```python
from build123d import *

# Parameters (mm, degrees)
F4_DEPTH = 25.4
F5_W     = 25.4
F5_H     = 25.4
F6_DEPTH = 76.2
F7_W     = 25.4
F7_H     = 25.4
F8_DEPTH = 88.9


# Not quite as in the source:
# - a variable given as a bare number and used for a length is read in inches; the dataset says mm whatever the document's units were


with BuildPart() as f4:
    # F3 (on Front) → F4 (new body)
    with BuildSketch(Plane.XZ):
        Polygon((0, 25.4), (0, 0), (25.4, 0), (101.6, 0), (101.6, 25.4), (25.4, 25.4), (25.4, 63.5), (0, 63.5), align=None)
    extrude(amount=-F4_DEPTH)

    # F5 (on face) → F6 (join)
    with BuildSketch(Plane(origin=(0, 25.4, 0), x_dir=(-1, 0, 0), z_dir=(0, 1, 0))):
        with Locations((-12.7, 50.8)):
            Rectangle(F5_W, F5_H)
    extrude(amount=F6_DEPTH)

    # F7 (on face) → F8 (join)
    with BuildSketch(Plane(origin=(0, 25.4, 0), x_dir=(-1, 0, 0), z_dir=(0, 1, 0))):
        with Locations((-88.9, 12.7)):
            Rectangle(F7_W, F7_H)
    extrude(amount=F8_DEPTH)


solid = f4.part
```
Verification items for the finished model (mm, model axes). A direction names the side the tool comes from. Coordinates: 2 decimals unless noted, no trailing zeros. Loops run counter-clockwise (first coordinate to the right, second up) from the corner with the lowest first, then second, coordinate; pieces in that order, holes last. Notation, with made-up numbers: (26, -31.75) - (33, -31.75) arc R29 cw to (33, -3.75) - close; hole circle Ø2 at (69.5, -2.75). An arc over 180 degrees is marked (long way). Put each result on its own line as item: value.
Item 1: Section check A-A (y = 37). Enter the section's corners in (x, z), then the cut area to 3 significant figures.
Conclusion:
outline: (0, 38.1) - (25.4, 38.1) - (25.4, 63.5) - (0, 63.5) - close; (76.2, 0) - (101.6, 0) - (101.6, 25.4) - (76.2, 25.4) - close
area: 1,290 mm2
Item 2: Section check B-B (x = 13.5). Enter the section's corners in (y, z), then the cut area to 3 significant figures.
Conclusion:
outline: (0, 0) - (25.4, 0) - (25.4, 38.1) - (101.6, 38.1) - (101.6, 63.5) - (0, 63.5) - close
area: 3,550 mm2
Item 3: Section check D-D (y = 18.5). Enter the section's corners in (x, z), then the cut area to 3 significant figures.
Conclusion:
outline: (0, 0) - (101.6, 0) - (101.6, 25.4) - (25.4, 25.4) - (25.4, 63.5) - (0, 63.5) - close
area: 3,550 mm2
Item 4: Scan lines: line 1 along Z through (x, y) = (83.5, 9.5); line 2 along X through (y, z) = (59.5, 7.5). Record each from-to range of solid material in increasing order.
Conclusion:
line 1: z = 0 to 25.4
line 2: x = 76.2 to 101.6
Item 5: Gauge pin test, flat ends, axial feed: pin 1 Ø7.5 at (x, y) = (11.5, 67.5) entering from -Z; pin 2 Ø10 at (y, z) = (29, 36.5) entering from +X; pin 3 Ø7.5 at (x, z) = (17.5, 49) entering from +Y; pin 4 Ø1 at (x, z) = (85.5, 27) entering from +Y. Record the tip position at first contact, or that the pin passes through.
Conclusion:
pin 1: stops at z = 38.1
pin 2: stops at x = 25.4
pin 3: stops at y = 101.6
pin 4: passes through
Item 6: Set-up check for faces 1 (the face through (13, 63, 38.1)), 2 (the face through (13, 50, 63.5)), 3 (the face through (76.2, 69, 13)), 4 (the face through (25.4, 50, 48)), 5 (the face through (38, 25.4, 15)): record each of +Z, -Z, +X, -X, +Y, -Y from which the full face is reachable in a straight line by a thin tool's end or side.
Conclusion:
face 1: -Z, +X, -X, +Y
face 2: +Z, +X, -X, +Y, -Y
face 3: +Z, -Z, -X, +Y
face 4: +Z, +X, +Y, -Y
face 5: -Z, -X, +Y
Item 7: Section check C-C (z = 29). Enter the section's corners in (x, y).
Conclusion:
outline: (0, 0) - (25.4, 0) - (25.4, 25.4) - (0, 25.4) - close
